Could you check a few things on this model? Use its own coordinates, in mm. Face numbers are marked on the shaded views. A direction names the side the tool comes from. Round coordinates to 2 decimals unless told otherwise and drop trailing zeros. Write each loop counter-clockwise with the first axis right and the second up, starting at its lowest first coordinate (ties: lowest second). Pieces come first, ordered by that corner, then holes.
```python
from build123d import *

# Parameters (mm, degrees)
SKETCH_R    = 20
PAD_DEPTH   = 10
SKETCH001_R = 17.5
SKETCH002_R = 17.45
SKETCH003_R = 15
SKETCH004_R = 14.95


with BuildPart() as part:
    # Sketch → Pad (new body)
    with BuildSketch(Plane.XY):
        Circle(SKETCH_R)
    extrude(amount=-PAD_DEPTH)

    # Sketch001 → AdditiveLoft section 0
    with BuildSketch(Plane.XY):
        Circle(SKETCH001_R)
    # Sketch002 (on DatumPlane) → AdditiveLoft section 1
    with BuildSketch(Plane.XY.offset(20)):
        Circle(SKETCH002_R)
    loft()

    # Sketch003 → SubtractiveLoft section 0
    with BuildSketch(Plane.XY):
        Circle(SKETCH003_R)
    # Sketch004 (on DatumPlane) → SubtractiveLoft section 1
    with BuildSketch(Plane.XY.offset(20)):
        Circle(SKETCH004_R)
    loft(mode=Mode.SUBTRACT)


solid = part.part
```
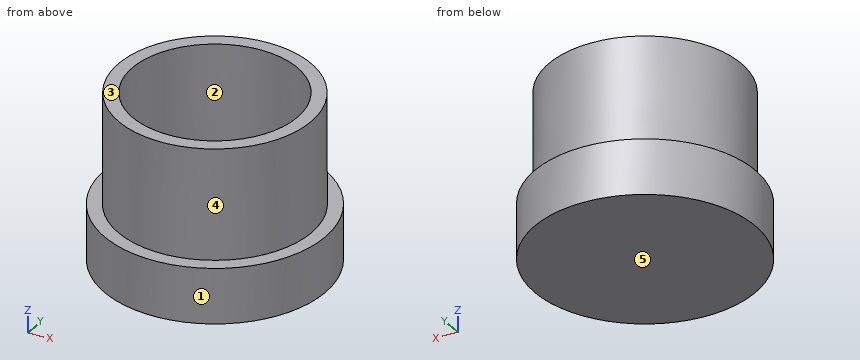
Q1. We'd pull the mould along X, two halves only. Please class the marked faces 1, 2 and 3: pulls with the +X half, pulls with the -X half, needs draft (parallel to the pull), parting line crosses it, or undercut.
Q2. Imagine slicing it at B-B, the plane z = 3. Write out the boundary of the cut face in (x, y) (1 decimal).
Q3. On a 3-axis mill with a long thin cutter (end or side, diameter ignored), from which of +Z, -Z, +X, -X, +Y, -Y can I reach the whole of each face in a straight line? I mean the marked faces 4 and 5. Say none if no direction works.
Q4. Imagine slicing it at C-C, the plane z = 10. Write out the boundary of the cut face in (x, y) (3 decimals).
Q5. If I drill on L1, parallel to Z at x = 12, y = -4; L2, parallel to Y at x = 8.5, z = 11.5; L3, parallel to Y at x = 0.5, z = -5, over which ranges is the centre line in solid material (lowest first)?
Q6. I'm going to push flat-ended pins straight in: pin 1 Ø4 at (x, y) = (5.5, 11.5) entering from +Z; pin 2 Ø5 at (x, z) = (3.5, 1) entering from +Y; pin 3 Ø1 at (y, z) = (4, 6) entering from +X; pin 4 Ø24 at (x, y) = (5, 4.5) entering from +Z. Where does each tip first touch, or does it pass through?
Q7. Imagine slicing it at A-A, the plane z = -8. Write out the boundary of the cut face in (x, y).
Results found:
1. face 1: parting line crosses it
1. face 2: undercut
1. face 3: needs draft
2. outline: circle Ø35 at (0, 0); hole circle Ø30 at (0, 0)
3. face 4: +Z
3. face 5: -Z, +X, -X, +Y, -Y
4. outline: circle Ø34.95 at (0, 0); hole circle Ø29.95 at (0, 0)
5. L1: z = -10 to 0
5. L2: y = -15.26 to -12.32, 12.32 to 15.26
5. L3: y = -19.99 to 19.99
6. pin 1: stops at z = 0
6. pin 2: stops at y = 19.96
6. pin 3: stops at x = 17.13
6. pin 4: stops at z = 20
7. outline: circle Ø40 at (0, 0)
